The listing builds one solid part. Answer for the finished solid, in the listing's coordinates (mm). A direction names the side the tool comes from. Round coordinates to 2 decimals unless told otherwise and drop trailing zeros. Write each loop counter-clockwise with the first axis right and the second up, starting at its lowest first coordinate (ties: lowest second). Pieces come first, ordered by that corner, then holes. Notation, with made-up numbers: M 36.5,26.25 L 52.5,26.25 A18 ccw 52.5,51.25 Z; hole C 67.5,0 d9. An arc over 180 degrees is marked long. Put each result on its own line as item: value. Start each with the question number.
```python
from build123d import *

# Parameters (mm, degrees)
SKETCH1_W           = 60
SKETCH1_H           = 40
SKETCH1_R           = 2.5
BOSS_EXTRUDE1_DEPTH = 10
SKETCH4_R           = 5
CUT_EXTRUDE1_DEPTH  = 5


with BuildPart() as part:
    # Sketch1 → Boss-Extrude1 (new body)
    with BuildSketch(Plane(origin=(0, 0, 0), x_dir=(1, 0, 0), z_dir=(0, 1, 0))):
        with Locations((30, -20)):
            Rectangle(SKETCH1_W, SKETCH1_H)
        with Locations(Location((51.2, -20, 0), (0, 0, 270))):
            Circle(SKETCH1_R, mode=Mode.SUBTRACT)
        with Locations(Location((8.8, -20, 0), (0, 0, 90))):
            Circle(SKETCH1_R, mode=Mode.SUBTRACT)
        with Locations(Location((30, -27.5, 0), (0, 0, 270))):
            Circle(SKETCH1_R, mode=Mode.SUBTRACT)
        with Locations(Location((30, -12.5, 0), (0, 0, 90))):
            Circle(SKETCH1_R, mode=Mode.SUBTRACT)
    extrude(amount=BOSS_EXTRUDE1_DEPTH)

    # Sketch4 → Cut-Extrude1 (cut)
    with BuildSketch(Plane.XZ):
        with Locations(Location((30, 27.5, 0), (0, 0, 270))):
            Circle(SKETCH4_R)
        with Locations(Location((30, 12.5, 0), (0, 0, 270))):
            Circle(SKETCH4_R)
    extrude(amount=-CUT_EXTRUDE1_DEPTH, mode=Mode.SUBTRACT)


solid = part.part
```
Item 1: Flat-ended cylindrical pins translate along their axes: pin 1 (3 mm diameter, centred on x = 8.8, z = 20, fed in from -Y); pin 2 (8 mm diameter, centred on x = 30, z = 12.5, fed in from -Y). Find the tip coordinate at first contact, or state that the pin passes through.
Item 2: Section D-D (x = 51.2) is taken. Give the vertices of the cut face in (y, z).
Item 3: Which of the six approach directions +Z, -Z, +X, -X, +Y, -Y give full straight-line access (tool end or side, diameter ignored) to faces 4 (the flat face through (30, 5, 40)), 5 (the flat face through (29, 5, 30))?
Item 4: Consider line 1 along X through (y, z) = (7.9, 27.5); line 2 along Z through (x, y) = (30, 7.75); line 3 along X through (y, z) = (3.6, 12.5). Determine where each line is inside the solid, lowest interval first. Write a range as [from, to].
Item 5: Section C-C (z = 20) is taken. Give the vertices of the cut face in (x, y).
Item 6: Section B-B (x = 30) is taken. Give the vertices of the cut face in (y, z), and give its area (3 significant figures).
Item 7: Section A-A (z = 12.5) is taken. Give the vertices of the cut face in (x, y), and give its area (3 significant figures).
Item 8: Determine the mould class of faces 1 (the flat face through (30, 0, 20)), 2 (the cylindrical face through (25.564, 2.465, 10.193)), 3 (the flat face through (0, 5, 20)) for opening direction X: released by +X, released by -X, zero draft, split by the parting line, or undercut.
Output values:
1. pin 1: passes through
1. pin 2: stops at y = 5
2. outline: M 0,0 L 10,0 L 10,17.5 L 0,17.5 Z; M 0,22.5 L 10,22.5 L 10,40 L 0,40 Z
3. face 4: +Z, +X, -X, +Y, -Y
3. face 5: -Y
4. line 1: x = [0, 27.5], [32.5, 60]
4. line 2: z = [0, 10], [15, 25], [30, 40]
4. line 3: x = [0, 25], [35, 60]
5. outline: M 0,0 L 6.3,0 L 6.3,10 L 0,10 Z; M 11.3,0 L 48.7,0 L 48.7,10 L 11.3,10 Z; M 53.7,0 L 60,0 L 60,10 L 53.7,10 Z
6. outline: M 0,0 L 10,0 L 10,10 L 5,10 L 5,7.5 L 0,7.5 Z; M 0,17.5 L 5,17.5 L 5,15 L 10,15 L 10,25 L 5,25 L 5,22.5 L 0,22.5 Z; M 0,32.5 L 5,32.5 L 5,30 L 10,30 L 10,40 L 0,40 Z
6. area: 250 mm^2
7. outline: M 0,0 L 25,0 L 25,5 L 27.5,5 L 27.5,10 L 0,10 Z; M 32.5,5 L 35,5 L 35,0 L 60,0 L 60,10 L 32.5,10 Z
7. area: 525 mm^2
8. face 1: zero draft
8. face 2: undercut
8. face 3: released by -X
